Autodesk Inventor part; units mm, degrees
ref_plane "Work Plane1" through (0, 6, -3.5) normal (0, 1, 0) x (-1, 0, 0)
ref_plane "Work Plane2" through (0, 2.5, -46) normal (0, 1, 0) x (-1, 0, 0)
ref_plane "YZ Plane" through (0, 0, 0) normal (1, 0, 0) x (0, 1, 0)
sketch "Sketch1" plane through (0, 0, 0) normal (1, 0, 0) x (0, 1, 0)
  line L0 (0, 0) -> (0, -92)
  line L1 (0, -92) -> (3.5, -92)
  line L2 (3.5, -92) -> (3.5, 0)
  line L3 (3.5, 0) -> (0, 0)
  line L4 (3.5, 0) -> (3.5, -6)
  line L5 (3.5, -92) -> (3.5, -86)
  line L6 (3.5, -92) -> (6, -92)
  line L7 (6, -92) -> (6, -86)
  line L8 (6, -86) -> (3.5, -86)
  line L9 (3.5, 0) -> (6, 0)
  line L10 (6, 0) -> (6, -6)
  line L11 (6, -6) -> (3.5, -6)
  line L12 (3.5, -86) -> (0.5, -86)
  line L13 (0.5, -86) -> (0.5, -6)
  line L14 (0.5, -6) -> (3.5, -6)
  line L15 (6, -6) -> (6, -7)
  line L16 (6, -7) -> (0.5, -7)
  line L17 (6, -86) -> (6, -85)
  line L18 (6, -85) -> (0.5, -85)
  line L19 (3.5, -7) -> (3.6267, -7)
  line L20 (2.5, -7) -> (2.5, -85)
  line L21 (0.5, -6) -> (0.5, -36)
  line L22 (0.5, -36) -> (0.75, -36)
  line L23 (0.75, -36) -> (0.75, -86)
  line L24 (0.75, -86) -> (0, -86)
  point P0 (3.5, -85)
  point P1 (2, -6)
  point P2 (3.6267, -85)
  dimension "d0" = 92
  dimension "d1" = 3.5
  dimension "d2" = 6
  dimension "d3" = 6
  dimension "d5" = 2.5
  dimension "d6" = 2.5
  dimension "d7" = 3
  dimension "d8" = 1
  dimension "d9" = 1
  dimension "d22" = 2
  dimension "d41" = 30
  dimension "d42" = 0.25
  dimension "d43" = 50
revolve "Revolution1" add sketch "Sketch1" angle 360 about axis through (0, 0, 0) along (0, 0, -1) contours L9 L10 L11 L2 | L11 L15 L16 L2 | L2 L16 L13 L14 | L2 L8 L7 L6 | L23 L18 L2 L12 | L2 L18 L17 L8 | L23 L22 L13 L16 L20 L18
thread "Thread1"
thread "Thread2"
chamfer "Chamfer1" distance 0.5 angle 45 2 edges at (0, -3.5, 0) (0, -3.5, -92)
chamfer "Chamfer2" distance 0.5 angle 45 4 edges at (0, -6, -92) (0, -6, -85) (0, -6, -7) (0, -6, 0)
chamfer "Chamfer3" distance 3 angle 45 2 edges at (0, -2.5, -7) (0, -2.5, -85)
ref_plane "Work Plane1" through (0, 6, -3.5) normal (0, 1, 0) x (-1, 0, 0)
ref_plane "Work Plane2" through (0, 2.5, -46) normal (0, 1, 0) x (-1, 0, 0)
sketch "Sketch2" plane through (0, 6, -3.5) normal (0, 1, 0) x (-1, 0, 0)
  point P0 (0, 3.5)
  point P1 (0, 0)
  point P2 (0, 0)
sketch "Sketch3" plane through (0, 2.5, -46) normal (0, 1, 0) x (-1, 0, 0)
  point P0 (0, 46)
  point P1 (0, 0)
hole "Hole1" at (0, 6, -3.5) direction (0, -1, 0) diameter 1 depth 0.5 tip angle 118
hole "Hole2" at (0, 2.5, -46) direction (0, -1, 0) diameter 1 depth 0.5 tip angle 118
properties part number "Heater"
Check sheet for the modelled part. Datum: model origin and axes. Units: mm. A direction names the side the tool comes from. Coordinates: 2 decimals unless noted, no trailing zeros. Write each loop counter-clockwise with the first axis right and the second up, starting at its lowest first coordinate (ties: lowest second). Pieces come first, ordered by that corner, then holes. Notation, with made-up numbers: (9, -32.5) - (28, -32.5) arc R12 ccw to (28, -22.5) - close; hole circle Ø9 at (-4, -5). An arc over 180 degrees is marked (long way). One line per question, with ' | ' between items.
Item 1: Access from +Z, -Z, +X, -X, +Y, -Y to the whole of each face (thin tool, end or side, straight path). Record for faces 1 (the face through (-2, -4, 0)), 2 (the face through (1.341, 3.233, -88.712)), 3 (the face through (2.624, -0.583, -9.812)), 4 (the face through (1.341, 3.233, -3.212)).
Determined:
face 1: +Z, +X, -X, +Y, -Y | face 2: -Z | face 3: none | face 4: +Z
Item 2: Thickness scan on line 1 (X direction, y = 0, z = -4.75); line 2 (Z direction, x = 0, y = 5.75); line 3 (X direction, y = 0, z = -27). Record the ranges inside material, lowest first. Write a range as [from, to].
Determined:
line 1: x = [-6, -3.5], [3.5, 6] | line 2: z = [-91.75, -85.25], [-6.75, -4], [-3, -0.25] | line 3: x = [-2.5, -0.5], [0.5, 2.5]
Item 3: Mould release check, pull along X, two halves, no side actions. Record for faces 5 (the face through (0.03, -0.75, -61.35)), 6 (the face through (-2, -4, -92)), 7 (the face through (-2.44, -0.54, -46.5)): pulls with the +X half, pulls with the -X half, needs draft (parallel to the pull), parting line crosses it, or undercut.
Determined:
face 5: undercut | face 6: needs draft | face 7: parting line crosses it
Item 4: Gauge pin test, flat ends, axial feed: P1, Ø5.5, axis at x = -1.5, y = 0.5, coming from the -Z side; P2, Ø1.2, axis at x = 0, y = 0, coming from the +Z side; P3, Ø6, axis at x = -0.5, z = -75.5, coming from the -Y side; P4, Ø6, axis at y = 1, z = -17.5, coming from the -X side. Record the tip position at first contact, or that the pin passes through.
Determined:
P1: stops at z = -92 | P2: stops at z = -6 | P3: stops at y = -2.5 | P4: stops at x = -2.5
Item 5: Sectioned sample at A-A on z = -43.5. Record the boundary of the cut face in (x, y), plus the area to 3 significant figures.
Determined:
outline: circle Ø5 at (0, 0); hole circle Ø1.5 at (0, 0) | area: 17.9 mm2
